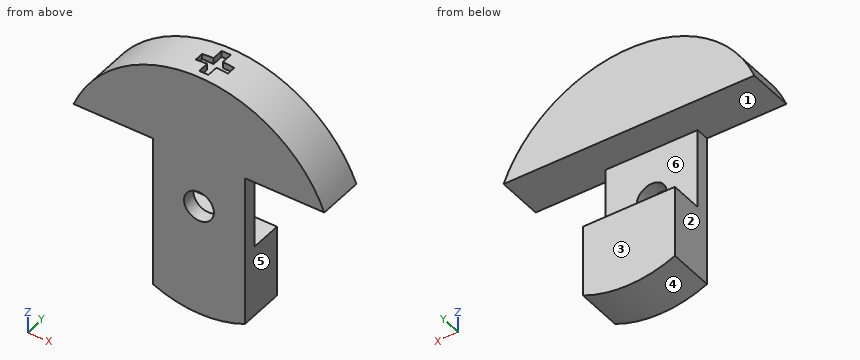
```python
from build123d import *

# Parameters (mm, degrees)
F1_DEPTH = 4
F2_W     = 2.83
F2_H     = 7
F3_DEPTH = 12.5
F6_DEPTH = 0.8
F7_R     = 1.3
F8_DEPTH = 4.001


with BuildPart() as f1:
    # F0 (on Front) → F1 (new body)
    with BuildSketch(Plane.XZ):
        with BuildLine():
            Line((-4, 4.37), (-4, -8.89171))
            ThreePointArc((-4, -8.89171), (0, -9.75), (4, -8.89171))
            Line((4, -8.89171), (4, 4.37))
            Line((4, 4.37), (10.907135, 4.37))
            ThreePointArc((10.907135, 4.37), (0, 11.75), (-10.907135, 4.37))
            Line((-10.907135, 4.37), (-4, 4.37))
        make_face()
    extrude(amount=F1_DEPTH)

    # F2 (on Right) → F3 (cut, symmetric)
    with BuildSketch(Plane.YZ):
        with Locations((-1.415, 0.87)):
            Rectangle(F2_W, F2_H)
    extrude(amount=F3_DEPTH, both=True, mode=Mode.SUBTRACT)

    # F5 (on offset) → F6 (cut)
    with BuildSketch(Plane.XY.offset(12)):
        Polygon((-0.4, -1.6), (-1.4, -1.6), (-1.4, -2.4), (-0.4, -2.4), (-0.4, -3.4), (0.4, -3.4), (0.4, -2.4), (1.4, -2.4), (1.4, -1.6), (0.4, -1.6), (0.4, -0.6), (-0.4, -0.6), align=None)
    extrude(amount=-F6_DEPTH, mode=Mode.SUBTRACT)

    # F7 (on face) → F8 (cut, through all)
    with BuildSketch(Plane.XZ.offset(4)):
        Circle(F7_R)
    extrude(amount=-F8_DEPTH, mode=Mode.SUBTRACT)


solid = f1.part
```
Could you check a few things on this model? Use its own coordinates, in mm. Face numbers are marked on the shaded views. A direction names the side the tool comes from. Round coordinates to 2 decimals unless told otherwise and drop trailing zeros. Loops run counter-clockwise (first coordinate to the right, second up) from the corner with the lowest first, then second, coordinate; pieces in that order, holes last. Notation, with made-up numbers: (46.5, -34.75) - (55.5, -34.75) arc R19 ccw to (55.5, -19.75) - close; hole circle Ø2 at (62, 31.5). An arc over 180 degrees is marked (long way). Use CSV: the item, a comma, the result in double quotes.
Item 1: If we section it at B-B on z = 0: List the corners of the cut face in (x, y) for me.
Here are the results:
outline,"(-4, -4) - (-1.3, -4) - (-1.3, -2.83) - (-4, -2.83) - close; (1.3, -4) - (4, -4) - (4, -2.83) - (1.3, -2.83) - close"
Item 2: For the marked faces 1, 2 and 3, which set-ups out of +Z, -Z, +X, -X, +Y, -Y let a thin tool reach every point of the face, with its end or its side?
Here are the results:
face 1,"+Y"
face 2,"-Z, -X, +Y, -Y"
face 3,"+Z, -Z, +X, -X, +Y"
Item 3: If we section it at D-D on x = -3.5: List the corners of the cut face in (y, z) for me.
Here are the results:
outline,"(-4, -9.1) - (0, -9.1) - (0, -2.63) - (-2.83, -2.63) - (-2.83, 4.37) - (0, 4.37) - (0, 11.22) - (-4, 11.22) - close"
Item 4: I need wall thicknesses on L1, parallel to Z at x = 0, y = -3.15; L2, parallel to Z at x = 0, y = -3.55; L3, parallel to X at y = -3.05, z = -5. Which ranges of each line are inside material? Lowest first, please. Write a range as [from, to].
Here are the results:
L1,"z = [-9.75, -1.3], [1.3, 11.2]"
L2,"z = [-9.75, -1.3], [1.3, 11.75]"
L3,"x = [-4, 4]"
Item 5: Will these pins go through, and if not, where does the flat tip stop? pin 1 (1.5 mm diameter, centred on y = -0.5, z = 7, fed in from +X); pin 2 (1.5 mm diameter, centred on x = -5.5, y = -2, fed in from -Z); pin 3 (4 mm diameter, centred on x = 0, z = 0, fed in from +Y).
Here are the results:
pin 1,"stops at x = 9.95"
pin 2,"stops at z = 4.37"
pin 3,"stops at y = -2.83"
Item 6: If we section it at C-C on z = -6: List the corners of the cut face in (x, y) for me, then the cut area to 3 significant figures.
Here are the results:
outline,"(-4, -4) - (4, -4) - (4, 0) - (-4, 0) - close"
area,"32.0 mm²"
Item 7: If we mould it in two halves opening along Z, with no side actions, what happens to the marked faces 4, 5 and 6? For each: pulls with the +Z half, pulls with the -Z half, needs draft (parallel to the pull), parting line crosses it, or undercut.
Here are the results:
face 4,"pulls with the -Z half"
face 5,"needs draft"
face 6,"undercut"
Item 8: If we section it at A-A on x = 0: List the corners of the cut face in (y, z) for me.
Here are the results:
outline,"(-4, -9.75) - (0, -9.75) - (0, -2.63) - (-2.83, -2.63) - (-2.83, -1.3) - (-4, -1.3) - close; (-4, 1.3) - (-2.83, 1.3) - (-2.83, 4.37) - (0, 4.37) - (0, 11.75) - (-0.6, 11.75) - (-0.6, 11.2) - (-3.4, 11.2) - (-3.4, 11.75) - (-4, 11.75) - close"
